Design review of the part shown in the three views and the two pictorial views. Dimensions are in mm from the part's minimum x, y and z. A direction names the side the tool comes from. Coordinates: 2 decimals unless noted, no trailing zeros. Write each loop counter-clockwise with the first axis right and the second up, starting at its lowest first coordinate (ties: lowest second). Pieces come first, ordered by that corner, then holes. Notation, with made-up numbers: (37.5, -13.75) - (70.5, -13.75) arc R13 ccw to (70.5, -4.75) - close; hole circle Ø1 at (60.5, 1.5). An arc over 180 degrees is marked (long way). Answer as CSV lines item,"result". Start each with the question number.
Q1. We need section B-B (z = 4.75). Write out the cut boundary in (x, y), plus the area to 3 significant figures.
Q2. For line 1 along Y through (x, z) = (1.5, 7.75); line 2 along X through (y, z) = (7.25, 5.5); line 3 along X through (y, z) = (4.25, 6.5), list the stretches that pass through material, from the lowest coordinate up. Write a range as [from, to].
Q3. We need section A-A (y = 6.5). Write out the cut boundary in (x, z), plus the area to 3 significant figures.
Q4. Clearance check with flat-ended pins moving along their axes: pin 1 (2 mm diameter, centred on x = 3, y = 4.5, fed in from +Z); pin 2 (2 mm diameter, centred on x = 7.5, y = 1.5, fed in from +Z); pin 3 (4 mm diameter, centred on y = 3.5, z = 2, fed in from -X). State where each tip first meets the part, or that it passes through.
Q5. Mouldability with a two-part tool opening along X and no side actions: class the marked faces 4, 5 and 6 as pulls with the +X half, pulls with the -X half, needs draft (parallel to the pull), parting line crosses it, or undercut.
Q6. We need section C-C (y = 1.25). Write out the cut boundary in (x, z).
Q7. Machinability: for the marked faces 1, 2 and 3, which of the approach directions +Z, -Z, +X, -X, +Y, -Y give a long, thin tool a straight path to every point of the face, cutting with its end or side? Answer none if there is none.
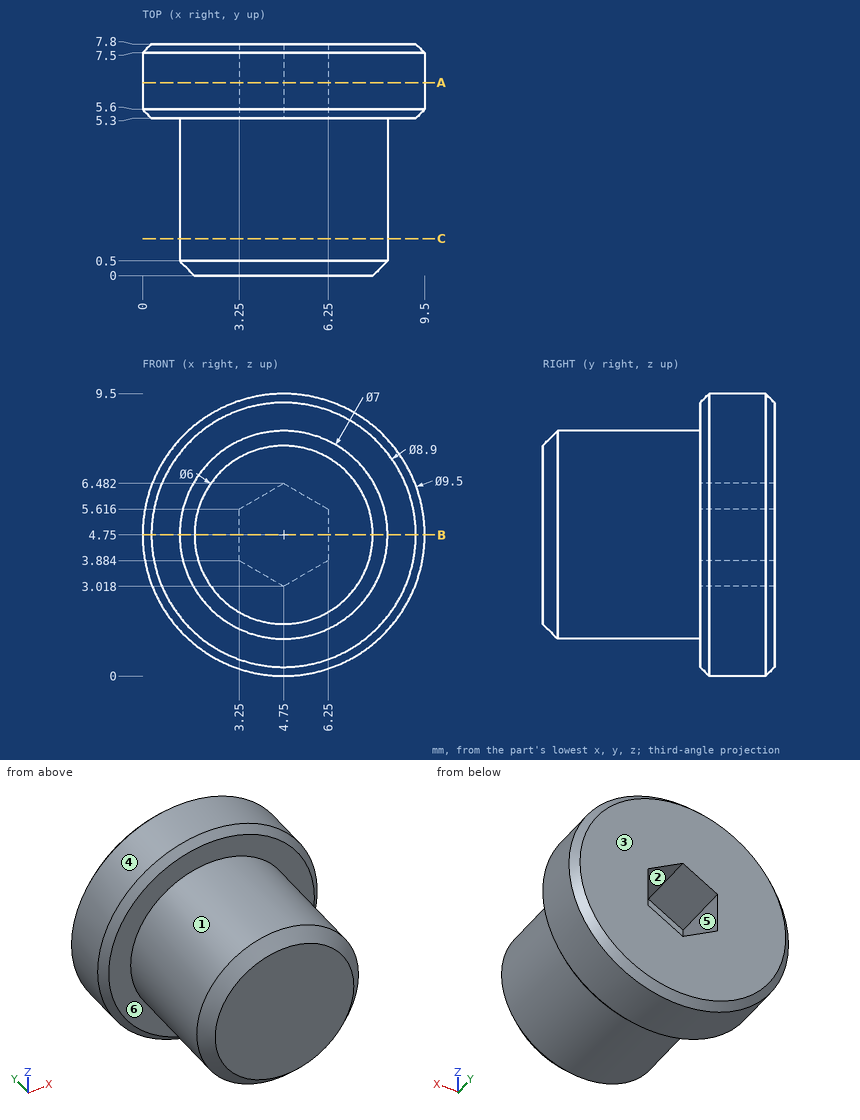
Results list:
1,outline,"(0, 5.6) - (0.3, 5.3) - (1.25, 5.3) - (1.25, 0.5) - (1.75, 0) - (7.75, 0) - (8.25, 0.5) - (8.25, 5.3) - (9.2, 5.3) - (9.5, 5.6) - (9.5, 7.5) - (9.2, 7.8) - (6.25, 7.8) - (6.25, 5.3) - (3.25, 5.3) - (3.25, 7.8) - (0.3, 7.8) - (0, 7.5) - close"
1,area,"52.9 mm2"
2,line 1,"y = [5.3, 7.8]"
2,line 2,"x = [0.06, 3.25], [6.25, 9.44]"
2,line 3,"x = [1.72, 7.78]"
3,outline,"circle Ø9.5 at (4.75, 4.75); hole (3.25, 3.88) - (4.75, 3.02) - (6.25, 3.88) - (6.25, 5.62) - (4.75, 6.48) - (3.25, 5.62) - close"
3,area,"63.1 mm2"
4,pin 1,"stops at z = 9.12"
4,pin 2,"stops at z = 7.78"
4,pin 3,"stops at x = 0.71"
5,face 4,"parting line crosses it"
5,face 5,"undercut"
5,face 6,"needs draft"
6,outline,"circle Ø7 at (4.75, 4.75)"
7,face 1,"-Y"
7,face 2,"+Y"
7,face 3,"+Z, -Z, +X, -X, +Y"
